```python
from build123d import *

# Parameters (mm, degrees)
F0_W     = 167.894
F0_H     = 200.025
F1_DEPTH = 90.805
F2_W     = 1.27
F2_H     = 7.4168746429
F2_W_2   = 5.461
F2_H_2   = 1.27
F3_DEPTH = 90.806
F4_T     = -16.51
F5_T     = -0.254


with BuildPart() as f1:
    # F0 (on Front) → F1 (new body)
    with BuildSketch(Plane.XZ):
        Rectangle(F0_W, F0_H)
    extrude(amount=F1_DEPTH)

    # F2 (on face) → F3 (cut, through all)
    with BuildSketch(Plane.XZ.offset(90.805)):
        Polygon((37.465, 100.0125), (-37.465, 100.0125), (-3.937, 76.5359416589), (1.524, 76.5359416589), align=None)
        Polygon((-40.9689176242, 3.7084373214), (-83.947, 65.0875), (-83.947, -65.0875), (-40.9689176242, -3.7084373214), align=None)
        Polygon((83.947, -51.9794289873), (83.947, 51.9794289873), (50.1472877587, 3.7084373214), (50.1472877587, -3.7084373214), align=None)
        Polygon((-1.9427287361, -81.3643829014), (-28.575, -100.0125), (30.1505425278, -100.0125), (3.5182712639, -81.3643829014), align=None)
        with Locations((-40.3339176242, 0)):
            Rectangle(F2_W, F2_H)
        with Locations((49.5122877587, 0)):
            Rectangle(F2_W, F2_H)
        with Locations((-1.2065, 75.9009416589)):
            Rectangle(F2_W_2, F2_H_2)
        with Locations((0.7877712639, -80.7293829014)):
            Rectangle(F2_W_2, F2_H_2)
    extrude(amount=-F3_DEPTH, mode=Mode.SUBTRACT)

    # F4
    f4_openings = [f1.faces().sort_by_distance(p)[0] for p in [
        (2.503833, -90.805, -1.127696),
    ]]
    offset(amount=F4_T, openings=f4_openings, kind=Kind.INTERSECTION)

    # F5
    f5_openings = [f1.faces().sort_by_distance(p)[0] for p in [
        (2.503833, 0, -1.127696),
    ]]
    offset(amount=F5_T, openings=f5_openings, kind=Kind.INTERSECTION)


solid = f1.part
```
Can you work these out from the model? Positions are in its coordinate system, mm. A direction names the side the tool comes from. Coordinates: 2 decimals unless noted, no trailing zeros. Loops run counter-clockwise (first coordinate to the right, second up) from the corner with the lowest first, then second, coordinate; pieces in that order, holes last. Notation, with made-up numbers: (56, 34) - (79, 34) arc R21 ccw to (79, 55) - close; hole circle Ø8 at (85.25, 44). An arc over 180 degrees is marked (long way). Use a Markdown table: item, result.
Item 1: If I drill on probe 1 along X at (y, z) = (-47, -72.5); probe 2 along X at (y, z) = (-64.5, 61); probe 3 along X at (y, z) = (-57, 5), over which ranges is the centre line in solid material (lowest first)? Write a range as from..to.
Numbers:
| item | result |
|---|---|
| probe 1 | x = -83.95..-83.69, -67.69..-67.44, -18.45..-18.2, 19.77..20.03, 67.44..67.69, 83.69..83.95 |
| probe 2 | x = -81.08..-80.77, -61.24..-60.93, -20.45..-20.19, 17.78..18.03, 67.44..67.69, 83.69..83.95 |
| probe 3 | x = -41.87..-41.56, -23.44..-23.19, 32.37..32.62, 50.74..51.05 |
Item 2: We'd pull the mould along X, two halves only. Please class faces 1 (the face through (17.02, -46.04, -90.82)), 2 (the face through (-61, -45, 100.012)), 3 (the face through (-62.16, -46.04, 33.97)): released by +X, released by -X, zero draft, split by the parting line, or undercut.
Numbers:
| item | result |
|---|---|
| face 1 | undercut |
| face 2 | zero draft |
| face 3 | released by -X |
Item 3: Will these pins go through, and if not, where does the flat tip stop? pin 1 (6 mm diameter, centred on x = -36.5, z = 19, fed in from +Y); pin 2 (1.5 mm diameter, centred on x = -37, z = 47.5, fed in from -Y); pin 3 (4 mm diameter, centred on y = -74, z = -6.5, fed in from +X).
Numbers:
| item | result |
|---|---|
| pin 1 | stops at y = -90.55 |
| pin 2 | stops at y = -16.51 |
| pin 3 | stops at x = 53.5 |
Item 4: I want a section at D-D on x = 10. Please give me the cut outline in (y, z) (3 decimals).
Numbers:
| item | result |
|---|---|
| outline | (-90.805, -85.903) - (0, -85.903) - (0, -85.593) - (-90.551, -85.593) - (-90.551, -63.838) - (-16.256, -63.838) - (-16.256, 59.01) - (-90.551, 59.01) - (-90.551, 81.769) - (0, 81.769) - (0, 82.072) - (-90.805, 82.072) - (-90.805, 58.756) - (-16.51, 58.756) - (-16.51, -63.584) - (-90.805, -63.584) - close |
Item 5: I want a section at B-B on y = -63.5. Give the number of separate pieces and of enclosed holes in the cut face, and give its area (3 significant figures).
Numbers:
| item | result |
|---|---|
| separate pieces | 2 |
| enclosed holes | 2 |
| area | 394 mm2 |
Item 6: For faces 4 (the face through (66.811, -46.038, -27.506)), 5 (the face through (67.691, -53, -71)), 6 (the face through (-51, -53, -83.502)), which set-ups out of +Z, -Z, +X, -X, +Y, -Y let a thin tool reach every point of the face, with its end or its side?
Numbers:
| item | result |
|---|---|
| face 4 | +X, +Y, -Y |
| face 5 | +Y |
| face 6 | -Y |
Item 7: I want a section at C-C on z = 28. Please give me the cut outline in (x, y) (3 decimals).
Numbers:
| item | result |
|---|---|
| outline | (-57.978, -90.805) - (-37.823, -90.805) - (-37.823, -16.51) - (47.001, -16.51) - (47.001, -90.805) - (67.156, -90.805) - (67.156, 0) - (66.846, 0) - (66.846, -90.551) - (47.312, -90.551) - (47.312, -16.256) - (-38.133, -16.256) - (-38.133, -90.551) - (-57.668, -90.551) - (-57.668, 0) - (-57.978, 0) - close |
